Print and shaded views of the part. All mm, measured from the part's lowest x, y and z. A direction names the side the tool comes from. Give positions to 0.01 mm unless a question says otherwise; leave off trailing zeros. Loops run counter-clockwise (first coordinate to the right, second up) from the corner with the lowest first, then second, coordinate; pieces in that order, holes last. Notation, with made-up numbers: M -32.5,72.25 L -21.5,72.25 A19 cw -21.5,77.25 Z; hole C 4,37 d7. An arc over 180 degrees is marked long. Answer as CSV lines item,"result".
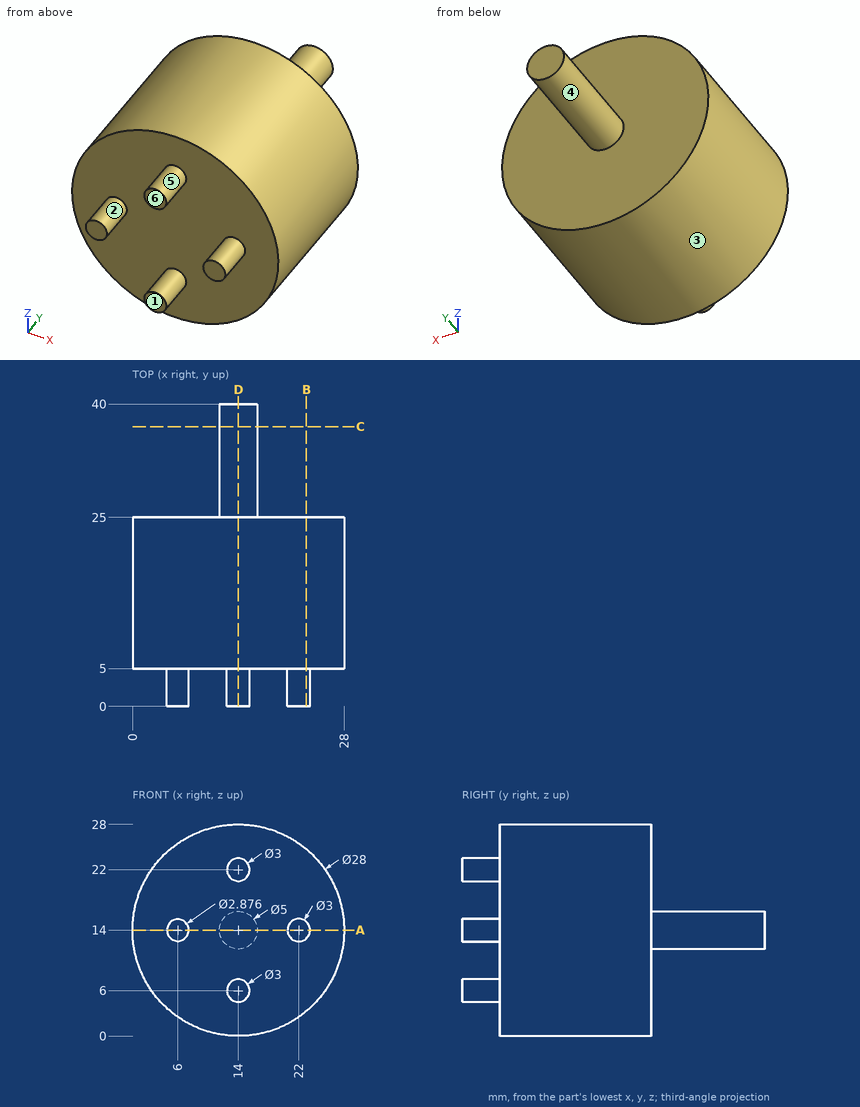
Q1. Which spindle directions (+Z, -Z, +X, -X, +Y, -Y) get a long thin tool onto all of the face, cutting with end or side? Do the marked faces 4, 5 and 6. Say none if no direction does.
Solution:
face 4,"+Y"
face 5,"-Y"
face 6,"+Z, -Z, +X, -X, -Y"
Q2. Pin check, flat tips, straight feed: P1, Ø6, axis at y = 17.5, z = 22, coming from the +X side; P2, Ø5, axis at x = 18, y = 10, coming from the +Z side; P3, Ø2, axis at x = 13.5, z = 6, coming from the +Y side. Stop position of each tip, or through.
Solution:
P1,"stops at x = 27.08"
P2,"stops at z = 27.92"
P3,"stops at y = 25"
Q3. Cut at D-D (x = 14). Write the cut outline in (y, z).
Solution:
outline,"M 0,4.5 L 5,4.5 L 5,0 L 25,0 L 25,11.5 L 40,11.5 L 40,16.5 L 25,16.5 L 25,28 L 5,28 L 5,23.5 L 0,23.5 L 0,20.5 L 5,20.5 L 5,7.5 L 0,7.5 Z"
Q4. Cut at B-B (x = 23). Write the cut outline in (y, z).
Solution:
outline,"M 0,12.88 L 5,12.88 L 5,3.28 L 25,3.28 L 25,24.72 L 5,24.72 L 5,15.12 L 0,15.12 Z"
Q5. Cut at A-A (z = 14). Write the cut outline in (x, y).
Solution:
outline,"M 0,5 L 4.56,5 L 4.56,0 L 7.44,0 L 7.44,5 L 20.5,5 L 20.5,0 L 23.5,0 L 23.5,5 L 28,5 L 28,25 L 16.5,25 L 16.5,40 L 11.5,40 L 11.5,25 L 0,25 Z"
Q6. Wall check: line 1 (Y direction, x = 19, z = 6.5); line 2 (Z direction, x = 12.5, y = 16); line 3 (X direction, y = 8.5, z = 5) (1 decimal). Give the ranges that are in metal, low to high. Write a range as [from, to].
Solution:
line 1,"y = [5, 25]"
line 2,"z = [0.08, 27.92]"
line 3,"x = [3.3, 24.7]"
Q7. Mould opens along X. For the marked faces 1, 2 and 3 say: released by +X, released by -X, zero draft, split by the parting line, or undercut.
Solution:
face 1,"zero draft"
face 2,"undercut"
face 3,"split by the parting line"
Q8. Cut at C-C (y = 37). Write the cut outline in (x, z), and give its area (3 significant figures).
Solution:
outline,"C 14,14 d5"
area,"19.6 mm²"
